For this review, take the finished solid that the model builds, in its own axes (mm). A direction names the side the tool comes from. Round coordinates to 2 decimals unless told otherwise and drop trailing zeros. Order: outer loops, then holes, each group sorted by start corner. A loop starts at its lowest first (then second) coordinate and runs counter-clockwise, first axis right, second up. Notation, with made-up numbers: (76, 47) - (121, 47) arc R18 ccw to (121, 53) - close; hole circle Ø6 at (47, 84.5). An arc over 180 degrees is marked (long way). One line per item, written item: value.
```python
from build123d import *

# Parameters (mm, degrees)
SKETCH_W        = 190
SKETCH_H        = 220
PAD_DEPTH       = 150
SKETCH001_W     = 178
SKETCH001_H     = 208
POCKET_DEPTH    = 147.5
SKETCH002_W     = 45
SKETCH002_H     = 85
SKETCH002_W_2   = 47.5
POCKET001_DEPTH = 100
SKETCH003_W     = 3
SKETCH003_H     = 11.5
POCKET002_DEPTH = 100
SKETCH004_W     = 15
SKETCH004_H     = 40
POCKET003_DEPTH = 150
SKETCH005_W     = 194.070648
SKETCH005_H     = 26.911476
POCKET004_DEPTH = 150.001
SKETCH006_W     = 2.43538
SKETCH006_H     = 10
SKETCH006_W_2   = 2.4
POCKET005_DEPTH = 173
SKETCH007_W     = 3.424065
SKETCH007_H     = 4
SKETCH007_W_2   = 3.834519
POCKET006_DEPTH = 173
SKETCH008_W     = 185.053348
SKETCH008_H     = 4
POCKET007_DEPTH = 173
PAD001_DEPTH    = 174
PAD002_DEPTH    = 174
POCKET008_DEPTH = 7
POCKET009_DEPTH = 200


with BuildPart() as part:
    # Sketch → Pad (new body)
    with BuildSketch(Plane.XY):
        with Locations((1.898805, 2.824203)):
            Rectangle(SKETCH_W, SKETCH_H)
    extrude(amount=PAD_DEPTH)

    # Sketch001 (on Face6 of Pad) → Pocket (cut)
    with BuildSketch(Plane.XY.offset(150)):
        with Locations((1.898805, 2.824203)):
            Rectangle(SKETCH001_W, SKETCH001_H)
    extrude(amount=-POCKET_DEPTH, mode=Mode.SUBTRACT)

    # Sketch002 (on Face4 of Pocket) → Pocket001 (cut)
    with BuildSketch(Plane(origin=(0, 0, 0), x_dir=(1, 0, 0), z_dir=(0, 0, -1))):
        with Locations((68.398805, -24.324203)):
            Rectangle(SKETCH002_W, SKETCH002_H)
        with Locations((-63.351195, -24.324203)):
            Rectangle(SKETCH002_W_2, SKETCH002_H)
    extrude(amount=-POCKET001_DEPTH, mode=Mode.SUBTRACT)

    # Sketch003 (on Face4 of Pocket001) → Pocket002 (cut)
    with BuildSketch(Plane(origin=(0, 0, 0), x_dir=(1, 0, 0), z_dir=(0, 0, -1))):
        with Locations((-19.601195, -7.074203)):
            Rectangle(SKETCH003_W, SKETCH003_H)
        with Locations((25.898805, -7.074203)):
            Rectangle(SKETCH003_W, SKETCH003_H)
    extrude(amount=-POCKET002_DEPTH, mode=Mode.SUBTRACT)

    # Sketch004 (on Face4 of Pocket002) → Pocket003 (cut)
    with BuildSketch(Plane(origin=(0, 0, 0), x_dir=(1, 0, 0), z_dir=(0, 0, -1))):
        with Locations((-85.601195, 87.175797)):
            Rectangle(SKETCH004_W, SKETCH004_H)
        with Locations((89.398805, 87.175797)):
            Rectangle(SKETCH004_W, SKETCH004_H)
    extrude(amount=-POCKET003_DEPTH, mode=Mode.SUBTRACT)

    # Sketch005 (on Face2 of Pocket003) → Pocket004 (cut, through all)
    with BuildSketch(Plane(origin=(0, 0, 0), x_dir=(1, 0, 0), z_dir=(0, 0, -1))):
        with Locations((-2.19445, 112.631535)):
            Rectangle(SKETCH005_W, SKETCH005_H)
    extrude(amount=-POCKET004_DEPTH, mode=Mode.SUBTRACT)

    # Sketch006 (on DatumPlane) → Pocket005 (cut)
    with BuildSketch(Plane.XZ.offset(67.175797)):
        with Locations((93.181115, 133.506973)):
            Rectangle(SKETCH006_W, SKETCH006_H)
        with Locations((-89.401195, 133.506973)):
            Rectangle(SKETCH006_W_2, SKETCH006_H)
    extrude(amount=-POCKET005_DEPTH, mode=Mode.SUBTRACT)

    # Sketch007 (on DatumPlane) → Pocket006 (cut)
    with BuildSketch(Plane.XZ.offset(67.175797)):
        with Locations((-87.572056, 133.506973)):
            Rectangle(SKETCH007_W, SKETCH007_H)
        with Locations((91.170921, 133.506973)):
            Rectangle(SKETCH007_W_2, SKETCH007_H)
    extrude(amount=-POCKET006_DEPTH, mode=Mode.SUBTRACT)

    # Sketch008 (on DatumPlane) → Pocket007 (cut)
    with BuildSketch(Plane.XZ.offset(67.175797)):
        with Locations((1.872131, 119.006973)):
            Rectangle(SKETCH008_W, SKETCH008_H)
    extrude(amount=-POCKET007_DEPTH, mode=Mode.SUBTRACT)

    # Sketch009 (on DatumPlane) → Pad001 (join)
    with BuildSketch(Plane.XZ.offset(67.175797)):
        Polygon((-87.101195, 117.006973), (-82.101195, 117.006973), (-87.101195, 112.006973), align=None)
        Polygon((90.898805, 117.006973), (85.898805, 117.006973), (90.898805, 112.006973), align=None)
    extrude(amount=-PAD001_DEPTH)

    # Sketch011 (on DatumPlane) → Pad002 (join)
    with BuildSketch(Plane.XZ.offset(67.175797)):
        Polygon((-87.101195, 150), (-82.101195, 150), (-87.101195, 146), align=None)
        Polygon((90.898805, 150), (90.898805, 146), (85.898805, 150), align=None)
    extrude(amount=-PAD002_DEPTH)

    # Sketch013 (on DatumPlane) → Pocket008 (cut)
    with BuildSketch(Plane.XY.offset(150)):
        with BuildLine():
            ThreePointArc((-87.098357, 62.824203), (-89.101195, 64.827042), (-91.104034, 62.824203))
            Line((-91.104034, 62.824203), (-91.104034, 59.41515))
            ThreePointArc((-91.104034, 59.41515), (-89.101195, 57.412311), (-87.098357, 59.41515))
            Line((-87.098357, 62.824203), (-87.098357, 59.41515))
        make_face()
        with BuildLine():
            ThreePointArc((-91.096694, -17.175797), (-89.101195, -19.171295), (-87.105697, -17.175797))
            Line((-87.105697, -17.175797), (-87.105697, -13.409031))
            ThreePointArc((-87.105697, -13.409031), (-89.101195, -11.413533), (-91.096694, -13.409031))
            Line((-91.096694, -17.175797), (-91.096694, -13.409031))
        make_face()
        with BuildLine():
            ThreePointArc((90.858933, -17.175797), (92.898805, -19.215669), (94.938676, -17.175797))
            Line((94.938676, -17.175797), (94.938676, -11.974619))
            ThreePointArc((94.938676, -11.974619), (92.898805, -9.934747), (90.858933, -11.974619))
            Line((90.858933, -17.175797), (90.858933, -11.974619))
        make_face()
        with BuildLine():
            ThreePointArc((94.89608, 62.824203), (92.898805, 64.821478), (90.901529, 62.824203))
            Line((90.901529, 62.824203), (90.901529, 57.425644))
            ThreePointArc((90.901529, 57.425644), (92.898805, 55.428369), (94.89608, 57.425644))
            Line((94.89608, 62.824203), (94.89608, 57.425644))
        make_face()
    extrude(amount=-POCKET008_DEPTH, mode=Mode.SUBTRACT)

    # Sketch019 (on Face6 of Pocket008) → Pocket009 (cut)
    with BuildSketch(Plane.YZ.offset(96.898805)):
        with BuildLine():
            ThreePointArc((-5.733227, 35.71838), (12.824203, 17.16095), (31.381633, 35.71838))
            Line((31.381633, 35.71838), (31.381633, 83.615097))
            ThreePointArc((31.381633, 83.615097), (12.824203, 102.172527), (-5.733227, 83.615097))
            Line((-5.733227, 35.71838), (-5.733227, 83.615097))
        make_face()
    extrude(amount=-POCKET009_DEPTH, mode=Mode.SUBTRACT)


solid = part.part
```
Item 1: Machinability: for faces 4 (the flat face through (-90.601, 18, 133)), 5 (the cylindrical face through (93.94, 13.23, 102.17)), 6 (the flat face through (94.896, 60, 147)), which of the approach directions +Z, -Z, +X, -X, +Y, -Y give a long, thin tool a straight path to every point of the face, cutting with its end or side? Answer none if there is none.
Returned:
face 4: -Y
face 5: +X, -X
face 6: +Z
Item 2: For P1, Ø2, axis at x = 93, y = 62.5, coming from the +Z side; P2, Ø4, axis at x = -61, z = 122, coming from the -Y side; P3, Ø3, axis at x = 93, z = 59, coming from the -Y side, all flat-tipped, find the tip position at first contact; note any pin that passes through.
Returned:
P1: z = 143
P2: y = 106.82
P3: y = -67.18
Item 3: Take a section at B-B (z = 43). Write out the cut boundary in (x, y).
Returned:
outline: (-93.1, -67.18) - (-87.1, -67.18) - (-87.1, -5.73) - (-93.1, -5.73) - close; (-93.1, 31.38) - (-87.1, 31.38) - (-87.1, 106.82) - (90.9, 106.82) - (90.9, 31.38) - (96.9, 31.38) - (96.9, 112.82) - (-93.1, 112.82) - close; (90.9, -67.18) - (96.9, -67.18) - (96.9, -5.73) - (90.9, -5.73) - close
Item 4: Take a section at C-C (z = 10). Write out the cut boundary in (x, y).
Returned:
outline: (-93.1, -67.18) - (-87.1, -67.18) - (-87.1, 106.82) - (90.9, 106.82) - (90.9, -67.18) - (96.9, -67.18) - (96.9, 112.82) - (-93.1, 112.82) - close
Item 5: The part is to be moulded in two halves that separate along X. For faces 1 (the flat face through (90, 19, 117.007)), 2 (the flat face through (1, 112.824, 74)), 3 (the flat face through (96.899, 42, 74)), say which applies: +X half, -X half, draft (parallel to the pull), parting line (faces both ways), or undercut.
Returned:
face 1: undercut
face 2: draft
face 3: +X half
Item 6: Take a section at D-D (y = 46.5). Count the separate pieces of the cut face and the enclosed holes in it, plus the area to 3 significant figures.
Returned:
separate pieces: 3
enclosed holes: 0
area: 1,970 mm^2
Item 7: Wall thickness on line 1 (X direction, y = 38, z = 81.5); line 2 (Y direction, x = -75.5, z = 137.5); line 3 (Z direction, x = 5.5, y = -54): over which ranges is each line inside the solid? List them lowest first.
Returned:
line 1: -93.1 to -87.1, 90.9 to 96.9
line 2: 106.82 to 112.82
line 3: 0 to 2.5
Item 8: Take a section at A-A (x = 48.5). Write out the cut boundary in (y, z).
Returned:
outline: (-99.18, 0) - (-18.18, 0) - (-18.18, 2.5) - (-99.18, 2.5) - close; (66.82, 0) - (112.82, 0) - (112.82, 150) - (106.82, 150) - (106.82, 2.5) - (66.82, 2.5) - close
